```python
from build123d import *

# Parameters (mm, degrees)
F0_R     = 14
F0_R_2   = 13.5
F1_DEPTH = 80
F2_W     = 26.356387
F2_H     = 11.70228
F3_DEPTH = 25.4
F4_W     = 26.242665
F4_H     = 11.610649
F5_DEPTH = 25.4


with BuildPart() as f1:
    # F0 (on Top) → F1 (new body)
    with BuildSketch(Plane.XY):
        Circle(F0_R)
        Circle(F0_R_2, mode=Mode.SUBTRACT)
    extrude(amount=F1_DEPTH)

    # F2 (on Front) → F3 (cut)
    with BuildSketch(Plane.XZ):
        with Locations((0.00854, 61.186025)):
            Rectangle(F2_W, F2_H)
    extrude(amount=-F3_DEPTH, mode=Mode.SUBTRACT)

    # F4 (on Front) → F5 (cut)
    with BuildSketch(Plane.XZ):
        with Locations((0.058447, 61.244421)):
            Rectangle(F4_W, F4_H)
    extrude(amount=F5_DEPTH, mode=Mode.SUBTRACT)


solid = f1.part
```
CAD build for the part. Positions are in the model's coordinates, mm. A direction names the side the tool comes from. Round coordinates to 2 decimals unless told otherwise and drop trailing zeros. Order: outer loops, then holes, each group sorted by start corner. A loop starts at its lowest first (then second) coordinate and runs counter-clockwise, first axis right, second up. Notation, with made-up numbers: (-19.75, 20) - (21.25, 20) arc R12 ccw to (21.25, 32) - close; hole circle Ø8 at (15, -13). An arc over 180 degrees is marked (long way). Answer in a Markdown table with one row per item. Add a question column.
(1) 3-axis set-ups, long thin cutter, end or side, ignore diameter. For faces 1 (the face through (-13.487, 0.594, 30.551)), 2 (the face through (-13.063, -4, 61)), 3 (the face through (-13.17, 4, 61)): which of +Z, -Z, +X, -X, +Y, -Y reach the whole face in a straight line?
(2) Drop flat-ended pins along their axis: pin 1 Ø12 at (x, z) = (-9.5, 32.5) entering from -Y; pin 2 Ø1 at (x, z) = (6, 23.5) entering from -Y; pin 3 Ø4 at (y, z) = (4.5, 39) entering from +X (3 decimals). Give the stop position or say it passes through.
(3) Band-saw the part on B-B on y = 0. List the corners of the cut face in (x, z), and give its area (3 significant figures).
(4) Band-saw the part on C-C on y = -9.25. List the corners of the cut face in (x, z), and give its area (3 significant figures).
(5) Band-saw the part on D-D on z = 24.5. List the corners of the cut face in (x, y).
(6) Band-saw the part on A-A on x = 0. List the corners of the cut face in (y, z).
(7) Probe L1, parallel to Y at x = 0, z = 28.5; L2, parallel to Z at x = -6.5, y = 12; L3, parallel to X at y = 4, z = 21. List the from-to ranges inside material, lowest first. Write a range as [from, to].
Data:
| question | item | result |
|---|---|---|
| 1 | face 1 | +Z, -Z |
| 1 | face 2 | +Y, -Y |
| 1 | face 3 | +Y |
| 2 | pin 1 | stops at y = -13.56 |
| 2 | pin 2 | stops at y = -12.87 |
| 2 | pin 3 | stops at x = 13.775 |
| 3 | outline | (-14, 0) - (-13.5, 0) - (-13.5, 80) - (-14, 80) - close; (13.5, 0) - (14, 0) - (14, 80) - (13.5, 80) - close |
| 3 | area | 80.0 mm^2 |
| 4 | outline | (-10.51, 0) - (-9.83, 0) - (-9.83, 55.44) - (-10.51, 55.44) - close; (-10.51, 67.05) - (-9.83, 67.05) - (-9.83, 80) - (-10.51, 80) - close; (9.83, 0) - (10.51, 0) - (10.51, 55.44) - (9.83, 55.44) - close; (9.83, 67.05) - (10.51, 67.05) - (10.51, 80) - (9.83, 80) - close |
| 4 | area | 92.5 mm^2 |
| 5 | outline | circle Ø28 at (0, 0); hole circle Ø27 at (0, 0) |
| 6 | outline | (-14, 0) - (-13.5, 0) - (-13.5, 55.44) - (-14, 55.44) - close; (-14, 67.05) - (-13.5, 67.05) - (-13.5, 80) - (-14, 80) - close; (13.5, 0) - (14, 0) - (14, 55.33) - (13.5, 55.33) - close; (13.5, 67.04) - (14, 67.04) - (14, 80) - (13.5, 80) - close |
| 7 | L1 | y = [-14, -13.5], [13.5, 14] |
| 7 | L2 | z = [0, 55.33], [67.04, 80] |
| 7 | L3 | x = [-13.42, -12.89], [12.89, 13.42] |
